```python
from build123d import *

# Parameters (mm, degrees)
F1_DEPTH  = 2.5
F2_T      = -2
F5_SIZE   = 1
F6_W      = 170
F6_H      = 5
F7_DEPTH  = 37.501
F9_W      = 2
F9_H      = 10.5037409129
F10_DEPTH = 6.3
F13_R     = 5
F14_DEPTH = 2.5
F17_D     = 6


with BuildPart() as f1:
    # F0 (on Front) → F1 (new body, symmetric)
    with BuildSketch(Plane.XZ):
        with BuildLine():
            Line((0, 10), (0, 0))
            Line((0, 0), (70, 0))
            Line((70, 0), (70, 10))
            Line((70, 10), (50, 10))
            ThreePointArc((50, 10), (46.4644660941, 11.4644660941), (45, 15))
            Line((45, 15), (45, 25))
            Line((45, 25), (35, 25))
            Line((35, 25), (35, 15))
            ThreePointArc((35, 15), (33.5355339059, 11.4644660941), (30, 10))
            Line((30, 10), (0, 10))
        make_face()
    extrude(amount=F1_DEPTH, both=True)

    # F2
    f2_openings = [f1.faces().sort_by_distance(p)[0] for p in [
        (35.933685, 2.5, 7.254637),
    ]]
    offset(amount=F2_T, openings=f2_openings)

    # F3 (on Front) → F4 (revolve)
    with BuildSketch(Plane.XZ):
        Polygon((40, 37.5), (40, 25), (43, 25), (43, 27), (42.5, 27), (42.5, 35.5), (43, 35.5), (43, 37.5), align=None)
    revolve(axis=Axis((40, 0, 31.25), (0, 0, 1)))

    # F5
    f5_edges = [f1.edges().sort_by_distance(p)[0] for p in [
        (37, 0, 37.5),
    ]]
    chamfer(f5_edges, length=F5_SIZE)

    # F6 (on Top) → F7 (intersect, through all)
    with BuildSketch(Plane.XY):
        with Locations((1.8975138664, 0)):
            Rectangle(F6_W, F6_H)
    extrude(amount=F7_DEPTH, mode=Mode.INTERSECT)

    # F9 (on offset) → F10 (cut)
    with BuildSketch(Plane.XY.offset(37.6)):
        with Locations((40, 0)):
            Rectangle(F9_W, F9_H)
    extrude(amount=-F10_DEPTH, mode=Mode.SUBTRACT)

    # F11: F1 across plane


with BuildPart() as f1_1:
    add(f1.part)
    add(f1.part.mirror(Plane.XY))

    # F12: F1 across plane


with BuildPart() as f1_2:
    add(f1_1.part)
    add(f1_1.part.mirror(Plane.YZ))

    # F13 (on Front) → F14 (join, symmetric)
    with BuildSketch(Plane.XZ):
        with Locations((-40, 0)):
            Circle(F13_R)
        with Locations((-15, 0)):
            Circle(F13_R)
    extrude(amount=F14_DEPTH, both=True)

    # F17 (through all)
    with Locations(Plane.XZ.offset(10)):
        with Locations((-40, 0), (-15, 0)):
            Hole(F17_D / 2)


solid = f1_2.part
```
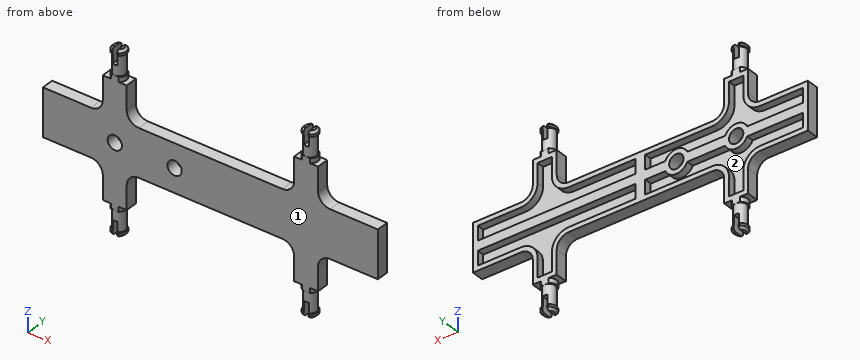
Here's how the part is built. I have some questions about the finished solid (model axes, mm). Face numbers are marked on the shaded views. Round coordinates to 2 decimals unless told otherwise and drop trailing zeros. Write each loop counter-clockwise with the first axis right and the second up, starting at its lowest first coordinate (ties: lowest second). Pieces come first, ordered by that corner, then holes. Notation, with made-up numbers: M 14.5,-11 L 60.5,-11 A11 ccw 60.5,-3 Z; hole C 67,14 d2. An arc over 180 degrees is marked long. Answer as CSV lines item,"result". Start each with the question number.
1. I need wall thicknesses on probe 1 along Z at (x, y) = (-15, 1.4); probe 2 along Z at (x, y) = (54.5, 0.65); probe 3 along X at (y, z) = (0.55, 5.5). Which ranges of each line are inside material? Lowest first, please.
2. Suppose I cut it at C-C on x = -48. Write out the boundary of the cut face in (y, z).
3. I'm going to push flat-ended pins straight in: pin 1 Ø0.9 at (y, z) = (1.5, -19.5) entering from -X; pin 2 Ø1.5 at (x, y) = (61.5, 1.5) entering from -Z; pin 3 Ø2.5 at (x, y) = (-14.5, -0.5) entering from +Z. Where does each tip first touch, or does it pass through?
4. Suppose I cut it at A-A on x = -15. Write out the boundary of the cut face in (y, z), then the cut area to 3 significant figures.
5. Thinking about a two-plate mould opening in Z: for the marked faces 1 and 2, which applies, released by +Z, released by -Z, zero draft, split by the parting line, or undercut?
6. Suppose I cut it at B-B on z = 0. Write out the boundary of the cut face in (x, y), then the cut area to 3 significant figures.
Check result:
1,probe 1,"z = -10 to -8, -5 to -3, 3 to 5, 8 to 10"
1,probe 2,"z = -10 to -8, -2 to 2, 8 to 10"
1,probe 3,"x = -70 to -68, -2 to 2, 68 to 70"
2,outline,"M -2.5,-10.42 L 2.5,-10.42 L 2.5,-8.29 L -0.5,-8.29 L -0.5,-2 L 2.5,-2 L 2.5,2 L -0.5,2 L -0.5,8.29 L 2.5,8.29 L 2.5,10.42 L -2.5,10.42 Z"
3,pin 1,"stops at x = -45"
3,pin 2,"stops at z = -10"
3,pin 3,"stops at z = 10"
4,outline,"M -2.5,-10 L 2.5,-10 L 2.5,-8 L -0.5,-8 L -0.5,-5 L 2.5,-5 L 2.5,-3 L -2.5,-3 Z; M -2.5,3 L 2.5,3 L 2.5,5 L -0.5,5 L -0.5,8 L 2.5,8 L 2.5,10 L -2.5,10 Z"
4,area,"52.0 mm2"
5,face 1,"zero draft"
5,face 2,"undercut"
6,outline,"M -70,-2.5 L -43,-2.5 L -43,2.5 L -70,2.5 Z; M -37,-2.5 L -18,-2.5 L -18,2.5 L -37,2.5 Z; M -12,-2.5 L 70,-2.5 L 70,2.5 L -12,2.5 Z"
6,area,"640 mm2"
